from build123d import *

# Parameters (mm, degrees)
SKETCH_1_W      = 60
SKETCH_1_H      = 60
EXTRUDE_1_DEPTH = 40
SKETCH_2_R      = 15
EXTRUDE_2_DEPTH = 30
SKETCH_3_R      = 15
EXTRUDE_3_DEPTH = 25
FILLET_11_R     = 5


with BuildPart() as part:
    # 草圖1 → 填料-伸長1 (new body)
    with BuildSketch(Plane(origin=(0, 0, 0), x_dir=(1, 0, 0), z_dir=(0, 1, 0))):
        Rectangle(SKETCH_1_W, SKETCH_1_H)
    extrude(amount=EXTRUDE_1_DEPTH)

    # 草圖2 → 填料-伸長2 (add)
    with BuildSketch(Plane.XZ):
        with Locations(Location((0, 0, 0), (0, 0, 270))):
            Circle(SKETCH_2_R)
    extrude(amount=EXTRUDE_2_DEPTH)

    # 草圖3 → 填料-伸長3 (add, symmetric)
    with BuildSketch(Plane(origin=(0, 0, 0), x_dir=(0, 0, -1), z_dir=(1, 0, 0))):
        with BuildLine():
            Line((-25, 40), (25, 40))
            Line((25, 40), (25, 56.698729811))
            ThreePointArc((25, 56.698729811), (0, 150), (-25, 56.698729811))
            Line((-25, 56.698729811), (-25, 40))
        make_face()
        with Locations((0, 100)):
            Circle(SKETCH_3_R, mode=Mode.SUBTRACT)
    extrude(amount=EXTRUDE_3_DEPTH, both=True)

    # 圓角11
    fillet_11_edges = [part.edges().sort_by_distance(p)[0] for p in [
        (-30, 40, 0),
        (0, 40, 30),
        (30, 40, 0),
        (0, 0, 30),
        (-30, 0, 0),
        (0, 0, -30),
        (30, 0, 0),
        (0, 40, -30),
        (30, 20, 30),
        (-30, 20, 30),
        (-30, 20, -30),
        (30, 20, -30),
    ]]
    fillet(fillet_11_edges, radius=FILLET_11_R - 0.0001)  # a hair under: the kernel refuses the full size


solid = part.part
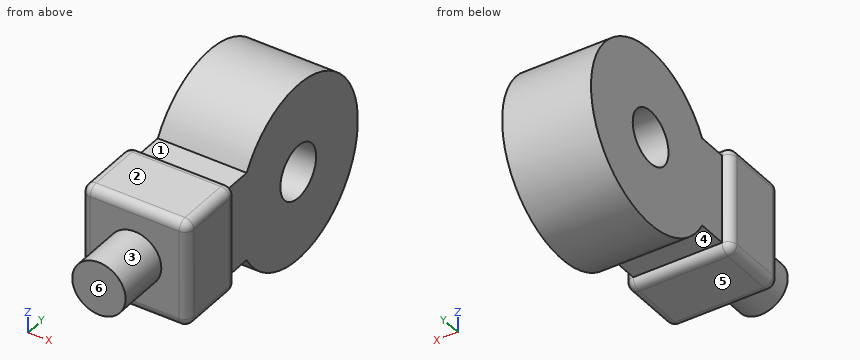
Build history of the part. All positions in model axes, mm. Face numbers are marked on the shaded views. A direction names the side the tool comes from. Give positions to 0.01 mm unless a question says otherwise; leave off trailing zeros. Loops run counter-clockwise (first coordinate to the right, second up) from the corner with the lowest first, then second, coordinate; pieces in that order, holes last. Notation, with made-up numbers: (-29.5, 73.5) - (5.5, 73.5) arc R12 ccw to (5.5, 85.5) - close; hole circle Ø10 at (58, -10.75). An arc over 180 degrees is marked (long way). Write item = value, one per line. Start each with the question number.
1) Tool access for the marked faces 1, 2 and 3: list every direction of +Z, -Z, +X, -X, +Y, -Y with a clear straight run to the whole face (end or side of a thin tool).
2) Band-saw the part on B-B on y = 100. Give the cut face in (x, z), plus the area to 3 significant figures.
3) Probe probe 1 along Y at (x, z) = (2, 0); probe 2 along Y at (x, z) = (-3, -6); probe 3 along X at (y, z) = (65.5, 2.5). List the from-to ranges inside material, lowest first. Write a range as from..to.
4) Drop flat-ended pins along their axis: pin 1 Ø4 at (x, y) = (-22.5, 59.5) entering from -Z; pin 2 Ø3 at (x, z) = (-3.5, 7.5) entering from +Y; pin 3 Ø10 at (x, y) = (-5.5, -11.5) entering from +Z. Give the stop position or say it passes through.
5) Band-saw the part on D-D on y = 20. Give the cut face in (x, z).
6) Pull direction Y, two halves, no side cores. Call the marked faces 4, 5 and 6: +Y half, -Y half, draft (parallel to the pull), parting line (faces both ways), or undercut.
Final values:
q1.face_1 = +Z, +X, -X
q1.face_2 = +Z, +X, -X, -Y
q1.face_3 = -Y
q2.outline = (-25, -50) - (25, -50) - (25, -15) - (-25, -15) - close; (-25, 15) - (25, 15) - (25, 50) - (-25, 50) - close
q2.area = 3,500 mm²
q3.probe_1 = -30..85, 115..150
q3.probe_2 = -30..86.25, 113.75..149.64
q3.probe_3 = -25..25
q4.pin_1 = -31.9
q4.pin_2 = 149.64
q4.pin_3 = 14.99
q5.outline = (-30, -25) arc R5 ccw to (-25, -30) - (25, -30) arc R5 ccw to (30, -25) - (30, 25) arc R5 ccw to (25, 30) - (-25, 30) arc R5 ccw to (-30, 25) - close
q6.face_4 = undercut
q6.face_5 = draft
q6.face_6 = -Y half
